Autodesk Inventor part; units mm, degrees
ref_plane "YZ Plane" through (0, 0, 0) normal (1, 0, 0) x (0, 1, 0)
ref_plane "XZ Plane" through (0, 0, 0) normal (0, 1, 0) x (-1, 0, 0)
ref_plane "XY Plane" through (0, 0, 0) normal (0, 0, 1) x (1, 0, 0)
sketch "Sketch1" plane through (0, 0, 0) normal (0, 1, 0) x (-1, 0, 0)
  point P0 (0, 0)
sketch "Sketch2" plane through (0, 0, 0) normal (0, 1, 0) x (-1, 0, 0)
  line L0 (-14.0823, -12.5349) -> (-51.0823, -12.5349)
  line L1 (-51.0823, -12.5349) -> (-51.0823, -57.4349)
  line L2 (-51.0823, -57.4349) -> (-14.0823, -57.4349)
  line L3 (-14.0823, -57.4349) -> (-14.0823, -12.5349)
  circle A0 centre (-32.5823, -34.9849) radius 30
  point P0 (0, 0)
  dimension "d0" = 37
  dimension "d1" = 44.9
extrude "Extrusion1" add sketch "Sketch2" against normal blind 1 contours L3 L2 L1 L0 | A0
extrude "Extrusion2" add sketch "Sketch2" along normal blind 22
sketch "Sketch3" plane through (32.5823, 22, -34.9849) normal (0, 1, 0) x (1, 0, 0)
  circle A0 centre (24.4505, 0.0199) radius 4.09
  point P0 (-32.5823, -34.9849)
  dimension "d9" = 8.18
extrude "Extrusion3" cut sketch "Sketch3" against normal up to next
sketch "Sketch4" plane through (32.5823, 22, -34.9849) normal (0, 1, 0) x (1, 0, 0)
  point P0 (-32.5823, -34.9849)
sketch "Sketch6" plane through (32.5823, 22, -34.9849) normal (0, 1, 0) x (1, 0, 0)
  circle A0 centre (0, 0) radius 30
  line L0 (-30, 0) -> (-24, 0)
  circle A1 centre (-24, 0) radius 2
  point P0 (-32.5823, -34.9849)
  dimension "d23" = 6
  dimension "d24" = 4
sketch "Sketch7" plane through (32.5823, 22, -34.9849) normal (0, 1, 0) x (1, 0, 0)
  circle A0 centre (0, 0) radius 30
  line L0 (0, -30) -> (0, -26.5)
  circle A1 centre (0, -26.5) radius 2
  line L1 (0, 30) -> (0, 26.5)
  circle A2 centre (0, 26.5) radius 2
  point P0 (-32.5823, -34.9849)
  dimension "d25" = 3.5
  dimension "d26" = 4
  dimension "d27" = 3.5
  dimension "d28" = 4
extrude "Extrusion5" cut sketch "Sketch7" against normal blind 10 contours A2 | A1
extrude "Extrusion6" cut sketch "Sketch6" against normal blind 10 contours A1
thread "Thread4"
thread "Thread5"
thread "Thread6"
sketch "Sketch8" plane through (32.5823, 22, -34.9849) normal (0, 1, 0) x (1, 0, 0)
  point P0 (-32.5823, -34.9849)
fillet "Fillet1" radius 2 1 edges at (62.5823, -1, -34.9849)
fillet "Fillet2" radius 5 4 edges at (14.0823, 11, -57.4349) (14.0823, 11, -12.5349) (51.0823, 11, -12.5349) (51.0823, 11, -57.4349)
sketch "Sketch10" plane through (0, -1, 0) normal (0, -1, 0) x (1, 0, 0)
  line L0 (38.5823, -44.9849) -> (26.5823, -44.9849)
  line L1 (26.5823, -44.9849) -> (26.5823, -24.9849)
  line L2 (26.5823, -24.9849) -> (38.5823, -24.9849)
  line L3 (38.5823, -24.9849) -> (38.5823, -44.9849)
  arc A0 (60.4997, -32.8347) -> (60.4961, -37.1806) centre (32.5823, -34.9849) ccw
  line L4 (38.5823, -44.9849) -> (26.5823, -24.9849) construction
  line L5 (26.5823, -44.9849) -> (38.5823, -24.9849) construction
  line L6 (43.6176, -37.4849) -> (40.1176, -37.4849)
  line L7 (40.1176, -37.4849) -> (40.1176, -32.4849)
  line L8 (40.1176, -32.4849) -> (43.6176, -32.4849)
  line L9 (43.6176, -32.4849) -> (43.6176, -37.4849)
  line L10 (43.6176, -37.4849) -> (40.1176, -32.4849) construction
  line L11 (40.1176, -37.4849) -> (43.6176, -32.4849) construction
  line L12 (25.1564, -37.4849) -> (21.6564, -37.4849)
  line L13 (21.6564, -37.4849) -> (21.6564, -32.4849)
  line L14 (21.6564, -32.4849) -> (25.1564, -32.4849)
  line L15 (25.1564, -32.4849) -> (25.1564, -37.4849)
  line L16 (25.1564, -37.4849) -> (21.6564, -32.4849) construction
  line L17 (21.6564, -37.4849) -> (25.1564, -32.4849) construction
  point P0 (0, 0)
  point P1 (41.8676, -34.9849)
  point P2 (23.4064, -34.9849)
  dimension "d49" = 12
  dimension "d50" = 20
  dimension "d51" = 3.5
  dimension "d52" = 5
  dimension "d53" = 3.5
  dimension "d54" = 5
extrude "Extrusion8" cut sketch "Sketch10" against normal blind 2
fillet "Fillet3" radius 1 2 edges at (32.5823, -1, -44.9849) (32.5823, -1, -24.9849)
properties part number "webcam_holder_center"
Input: part model. Units: mm. Frame: model coordinates. A direction names the side the tool comes from. Round coordinates to 2 decimals unless told otherwise and drop trailing zeros. Loops run counter-clockwise (first coordinate to the right, second up) from the corner with the lowest first, then second, coordinate; pieces in that order, holes last.
1) Section query A-A on y = 11.25. Return the cut outline in (x, z).
Ans:
outline: circle Ø60 at (32.58, -34.98); hole (14.08, -52.43) arc R5 ccw to (19.08, -57.43) - (46.08, -57.43) arc R5 ccw to (51.08, -52.43) - (51.08, -17.53) arc R5 ccw to (46.08, -12.53) - (19.08, -12.53) arc R5 ccw to (14.08, -17.53) - close; hole circle Ø8.18 at (57.03, -35)
2) Set-up query: faces 1 (the flat face through (13, 22, -35)), 2 (the flat face through (51.082, 11, -35)). Return all of +Z, -Z, +X, -X, +Y, -Y with unobstructed straight access to the full face (end or side cutting, diameter ignored); none if empty.
Ans:
face 1: +Z, -Z, +X, -X, +Y
face 2: +Y
3) Pin query (flat end, axial travel): pin 1 (6 mm diameter, centred on x = 25.5, z = -39, fed in from +Y); pin 2 (1.1 mm diameter, centred on x = 42, y = -0.5, fed in from +Z); pin 3 (0.8 mm diameter, centred on y = -0.5, z = -34, fed in from +X); pin 4 (11 mm diameter, centred on y = 6, z = -39, fed in from +X). Return the tip coordinate at first contact, or that it passes through.
Ans:
pin 1: stops at y = 0
pin 2: stops at z = -6.71
pin 3: stops at x = 62.27
pin 4: stops at x = 62.58
4) Pull-direction query (Z, two-part tool) for faces 3 (the flat face through (14.082, 11, -35)), 4 (the cylindrical face through (16.45, 11.32, -60.28)), 5 (the flat face through (39, -1, -35)), 6 (the cylindrical face through (52.947, 10.661, -35.185)); classes: released by +Z, released by -Z, zero draft, split by the parting line, or undercut.
Ans:
face 3: undercut
face 4: split by the parting line
face 5: zero draft
face 6: undercut
5) Section query B-B on y = 19.75. Return the cut outline in (x, z), plus the area to 3 significant figures.
Ans:
outline: circle Ø60 at (32.58, -34.98); hole circle Ø4 at (8.58, -34.98); hole (14.08, -52.43) arc R5 ccw to (19.08, -57.43) - (46.08, -57.43) arc R5 ccw to (51.08, -52.43) - (51.08, -17.53) arc R5 ccw to (46.08, -12.53) - (19.08, -12.53) arc R5 ccw to (14.08, -17.53) - close; hole circle Ø4 at (32.58, -61.48); hole circle Ø4 at (32.58, -8.48); hole circle Ø8.18 at (57.03, -35)
area: 1,100 mm2
6) Material intervals for line 1 (X direction, y = 17, z = -33.5); line 2 (Z direction, x = 31, y = 13); line 3 (Y direction, x = 23, z = -52), sorted ascending.
Ans:
line 1: x = 2.62 to 7.24, 9.92 to 14.08, 51.08 to 53.23, 60.84 to 62.55
line 2: z = -64.94 to -62.71, -60.26 to -57.43, -12.53 to -9.71, -7.26 to -5.03
line 3: y = -1 to 0
